from build123d import *

# Parameters (mm, degrees)
SKETCH1_R           = 11.1125
BOSS_EXTRUDE1_DEPTH = 11.049
SKETCH2_R           = 5.1562
BOSS_EXTRUDE2_DEPTH = 1.4986
SKETCH3_R           = 4.7625
BOSS_EXTRUDE5_DEPTH = 9.525
SKETCH4_R           = 3.937
BOSS_EXTRUDE6_DEPTH = 0.8382
SKETCH5_R           = 3.175
BOSS_EXTRUDE7_DEPTH = 22.225


with BuildPart() as part:
    # Sketch1 → Boss-Extrude1 (new body)
    with BuildSketch(Plane.XY):
        Circle(SKETCH1_R)
    extrude(amount=BOSS_EXTRUDE1_DEPTH)

    # Sketch2 → Boss-Extrude2 (add)
    with BuildSketch(Plane.XY.offset(11.049)):
        Circle(SKETCH2_R)
    extrude(amount=BOSS_EXTRUDE2_DEPTH)

    # Sketch3 → Boss-Extrude5 (add)
    with BuildSketch(Plane.XY.offset(11.049)):
        Circle(SKETCH3_R)
    extrude(amount=BOSS_EXTRUDE5_DEPTH)

    # Sketch4 → Boss-Extrude6 (add)
    with BuildSketch(Plane.XY.offset(20.574)):
        Circle(SKETCH4_R)
    extrude(amount=BOSS_EXTRUDE6_DEPTH)

    # Sketch5 → Boss-Extrude7 (add)
    with BuildSketch(Plane.XY.offset(11.049)):
        Circle(SKETCH5_R)
    extrude(amount=BOSS_EXTRUDE7_DEPTH)


solid = part.part
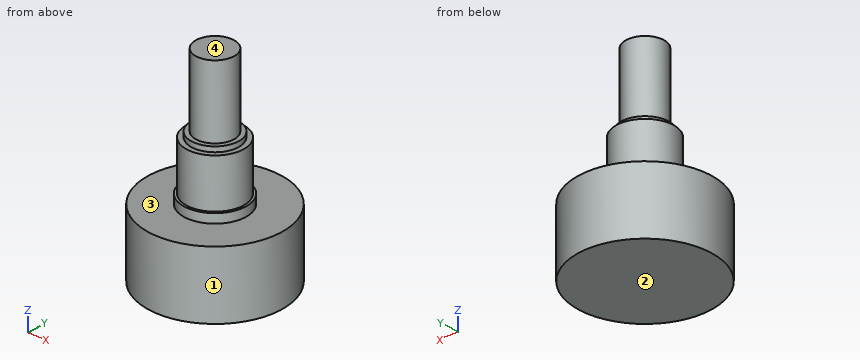
For this review, take the finished solid that the model builds, in its own axes (mm). Face numbers are marked on the shaded views. A direction names the side the tool comes from. Coordinates: 2 decimals unless noted, no trailing zeros. Order: outer loops, then holes, each group sorted by start corner. A loop starts at its lowest first (then second) coordinate and runs counter-clockwise, first axis right, second up. Notation, with made-up numbers: (9, -20) - (18, -20) arc R9 cw to (18, -10) - close; hole circle Ø5 at (89, 81). An arc over 180 degrees is marked (long way). Use one line per item in the form item = value.
Q1. For P1, Ø3, axis at x = -4.5, z = 7.5, coming from the +Y side; P2, Ø2, axis at x = 3, z = 29.5, coming from the -Y side; P3, Ø12, axis at y = -5.5, z = 7, coming from the -X side; P4, Ø10, axis at x = 7.5, z = 26, coming from the +Y side, all flat-tipped, find the tip position at first contact; note any pin that passes through.
Checked values:
P1 = 10.7
P2 = -2.47
P3 = -11.11
P4 = 1.96
Q2. Draft analysis for pull direction Y (two halves, no side actions). For the marked faces 1 and 2, state which applies: +Y half, -Y half, draft (parallel to the pull), parting line (faces both ways), or undercut.
Checked values:
face_1 = parting line
face_2 = draft
Q3. Consider section D-D (y = 6). Give the boundary of the cut face in (x, z).
Checked values:
outline = (-9.35, 0) - (9.35, 0) - (9.35, 11.05) - (-9.35, 11.05) - close
Q4. For the marked faces 3 and 4, list the 3-axis set-ups (+Z, -Z, +X, -X, +Y, -Y) from which the entire face can be reached by the end or side of a thin tool; tool diameter is ignored.
Checked values:
face_3 = +Z
face_4 = +Z, +X, -X, +Y, -Y
Q5. For probe 1 along Z at (x, y) = (-8.75, -2.25); probe 2 along Z at (x, y) = (4, -1.5); probe 3 along X at (y, z) = (-0.5, 30.5), list the stretches that pass through material, from the lowest coordinate up. Write a range as from..to.
Checked values:
probe_1 = 0..11.05
probe_2 = 0..20.57
probe_3 = -3.14..3.14
Q6. Consider section C-C (z = 13.5). Give the boundary of the cut face in (x, y) (1 decimal), then the cut area to 3 significant figures.
Checked values:
outline = circle Ø9.5 at (0, 0)
area = 71.3 mm2
